Autodesk Inventor part; units mm, degrees
ref_plane "YZ Plane" through (0, 0, 0) normal (1, 0, 0) x (0, 1, 0)
ref_plane "XZ Plane" through (0, 0, 0) normal (0, 1, 0) x (-1, 0, 0)
ref_plane "XY Plane" through (0, 0, 0) normal (0, 0, 1) x (1, 0, 0)
sketch "Szkic1" plane through (0, 0, 0) normal (0, 1, 0) x (-1, 0, 0)
  line L0 (0, 0) -> (42, 0)
  line L1 (42, 0) -> (42, -3)
  line L2 (42, -3) -> (0, -3)
  line L3 (0, -3) -> (0, 0)
  dimension "d0" = 42
  dimension "d1" = 3
extrude "Wyciągnięcie proste1" add sketch "Szkic1" along normal blind 8
sketch "Szkic2" plane through (0, 8, 0) normal (0, 1, 0) x (1, 0, 0)
  circle A0 centre (-38.7043, 1.357) radius 1
  point P0 (0, 0)
  dimension "d4" = 2
extrude "Wyciągnięcie proste2" cut sketch "Szkic2" against normal blind 0.2
sketch "Szkic3" plane through (-42, 0, 0) normal (0, 0, 1) x (1, 0, 0)
  line L0 (0, 8) -> (42, 8)
  line L1 (0, 8) -> (6, 8)
  line L2 (6, 0) -> (0, 0)
  line L3 (0, 0) -> (0, 8)
  line L4 (42, 0) -> (36, 0)
  line L5 (36, 8) -> (42, 8)
  line L6 (42, 8) -> (42, 0)
  circle A0 centre (9.5, 3) radius 0.6105
  line L7 (0, 0) -> (42, 0)
  circle A1 centre (18.5, 3) radius 0.61
  circle A2 centre (23.5, 3) radius 0.6105
  circle A3 centre (32.5, 3) radius 0.6105
  circle A4 centre (14, 3) radius 1.95
  circle A5 centre (28, 3) radius 1.95
  dimension "d7" = 6
  dimension "d8" = 8
  dimension "d9" = 6
  dimension "d10" = 1.221
  dimension "d11" = 3
  dimension "d12" = 1.22
  dimension "d13" = 1.221
  dimension "d14" = 1.221
  dimension "d15" = 3
  dimension "d16" = 3
  dimension "d17" = 3
  dimension "d18" = 9.5
  dimension "d19" = 9.5
  dimension "d20" = 9
  dimension "d21" = 9
  dimension "d22" = 3.9
  dimension "d23" = 3.9
  dimension "d24" = 3
  dimension "d25" = 4.5
  dimension "d26" = 4.5
  dimension "d27" = 3
extrude "Wyciągnięcie proste3" cut sketch "Szkic3" against normal blind 3 contours A0 | A1 | A2 | A3 | A4 | A5
properties part number "blmwall"
Geometry: final body of the model. Coordinates: model frame, mm. Coordinates: 2 decimals unless noted, no trailing zeros. Order: outer loops, then holes, each group sorted by start corner. A loop starts at its lowest first (then second) coordinate and runs counter-clockwise, first axis right, second up.
Item 1: Draft query along Y for faces 1 (the face through (-31.918, 3.183, -1.479)), 2 (the face through (0, 4, -2)), 3 (the face through (-22.918, 3.183, -1.479)), 4 (the face through (-39, 7.8, -1)). Return one class per face: released by +Y, released by -Y, zero draft, split by the parting line, or undercut.
Answer:
face 1: undercut
face 2: zero draft
face 3: undercut
face 4: released by +Y
Item 2: Material intervals for line 1 along X through (y, z) = (1.25, -2.2); line 2 along Y through (x, z) = (-18.5, -1.8); line 3 along Y through (x, z) = (-28, -2.05), sorted ascending.
Answer:
line 1: x = -42 to -28.86, -27.14 to -14.86, -13.14 to 0
line 2: y = 0 to 2.39, 3.61 to 8
line 3: y = 0 to 1.05, 4.95 to 8
Item 3: Contact query for a flat-ended pin moving along its axis: P1, Ø1.4, axis at x = -32.5, y = 3, coming from the -Z side. Output: stop coordinate, or through.
Answer:
P1: stops at z = -3
Item 4: Section query D-D (z = -0.9). Output: boundary loops of the cut face in (x, y), then the cut area to 3 significant figures.
Answer:
outline: (-42, 0) - (0, 0) - (0, 8) - (-37.81, 8) - (-37.81, 7.8) - (-39.59, 7.8) - (-39.59, 8) - (-42, 8) - close; hole circle Ø1.22 at (-32.5, 3); hole circle Ø3.9 at (-28, 3); hole circle Ø1.22 at (-23.5, 3); hole circle Ø1.22 at (-18.5, 3); hole circle Ø3.9 at (-14, 3); hole circle Ø1.22 at (-9.5, 3)
area: 307 mm2
Item 5: Section query C-C (x = -14). Output: boundary loops of the cut face in (y, z).
Answer:
outline: (0, -3) - (1.05, -3) - (1.05, 0) - (0, 0) - close; (4.95, -3) - (8, -3) - (8, 0) - (4.95, 0) - close
Item 6: Section query B-B (y = 3). Output: boundary loops of the cut face in (x, z).
Answer:
outline: (-42, -3) - (-33.11, -3) - (-33.11, 0) - (-42, 0) - close; (-31.89, -3) - (-29.95, -3) - (-29.95, 0) - (-31.89, 0) - close; (-26.05, -3) - (-24.11, -3) - (-24.11, 0) - (-26.05, 0) - close; (-22.89, -3) - (-19.11, -3) - (-19.11, 0) - (-22.89, 0) - close; (-17.89, -3) - (-15.95, -3) - (-15.95, 0) - (-17.89, 0) - close; (-12.05, -3) - (-10.11, -3) - (-10.11, 0) - (-12.05, 0) - close; (-8.89, -3) - (0, -3) - (0, 0) - (-8.89, 0) - close
Item 7: Section query A-A (x = -32.5). Output: boundary loops of the cut face in (y, z), then the cut area to 3 significant figures.
Answer:
outline: (0, -3) - (2.39, -3) - (2.39, 0) - (0, 0) - close; (3.61, -3) - (8, -3) - (8, 0) - (3.61, 0) - close
area: 20.3 mm2
